Can you work these out from the model? Positions are in its coordinate system, mm. A direction names the side the tool comes from. Give positions to 0.01 mm unless a question says otherwise; leave off trailing zeros. Loops run counter-clockwise (first coordinate to the right, second up) from the corner with the lowest first, then second, coordinate; pieces in that order, holes last. Notation, with made-up numbers: (37.25, 47.5) - (67.25, 47.5) arc R10 ccw to (67.25, 55.5) - close; hole circle Ø2 at (78, 75). An arc over 180 degrees is marked (long way). Answer as a JSON object with one key per item and string values. Group by question number.
Item 1: Which directions (+Z, -Z, +X, -X, +Y, -Y) give clear straight access to the entire face, cutting with the end or side of a thin tool? Please do faces 1 (the flat face through (-42, 25, -45)), 2 (the flat face through (-90, 62, -45)), 3 (the flat face through (-88, 90, -45)).
Item 2: Suppose I cut it at C-C on x = -61. Write out the boundary of the cut face in (y, z), and give its area (3 significant figures).
Item 3: Thinking about a two-plate mould opening in Y: for faces 4 (the flat face through (-72.075, 17.43, -45.49)), 5 (the flat face through (-28, 0, -45)), 6 (the cylindrical face through (-71.014, 84.297, -44.51)), 7 (the flat face through (-66, 34, -80)), which applies, pulls with the +Y half, pulls with the -Y half, needs draft (parallel to the pull), parting line crosses it, or undercut?
Item 4: Will these pins go through, and if not, where does the flat tip stop? pin 1 (6 mm diameter, centred on y = 27.5, z = -28.5, fed in from -X); pin 2 (22.5 mm diameter, centred on y = 45, z = -49, fed in from +X); pin 3 (3 mm diameter, centred on x = -57, z = -50.5, fed in from -Y).
Item 5: Suppose I cut it at B-B on y = 53.5. Write out the boundary of the cut face in (x, z).
Item 6: Suppose I cut it at A-A on z = -45. Write out the boundary of the cut face in (x, y).
Item 7: Suppose I cut it at D-D on y = 10.5. Count the separate pieces of the cut face and the enclosed holes in it, and give its area (3 significant figures).
Item 8: Please list where these lines run through material, in increasing order: L1, parallel to X at y = 66.5, z = -18; L2, parallel to Z at x = -74.5, y = 10.5; L3, parallel to Y at x = -43, z = -56.5.
from build123d import *

# Parameters (mm, degrees)
SKETCH1_W           = 90
SKETCH1_H           = 80
BOSS_EXTRUDE1_DEPTH = 90
SKETCH2_W           = 65
SKETCH2_H           = 65
CUT_EXTRUDE1_DEPTH  = 100
FILLET1_R           = 20
CUT_EXTRUDE2_DEPTH  = 100
SKETCH4_R           = 7.5
BOSS_EXTRUDE2_DEPTH = 150
SKETCH6_W           = 10
SKETCH6_H           = 127.279220614
CUT_EXTRUDE4_DEPTH  = 212.224744882


with BuildPart() as part:
    # Sketch1 → Boss-Extrude1 (new body)
    with BuildSketch(Plane(origin=(0, 0, 0), x_dir=(1, 0, 0), z_dir=(0, 1, 0))):
        with Locations((-45, 40)):
            Rectangle(SKETCH1_W, SKETCH1_H)
    extrude(amount=BOSS_EXTRUDE1_DEPTH)

    # Sketch2 → Cut-Extrude1 (cut)
    with BuildSketch(Plane(origin=(0, 0, -80), x_dir=(-1, 0, 0), z_dir=(0, 0, -1))):
        with Locations((32.5, 57.5)):
            Rectangle(SKETCH2_W, SKETCH2_H)
    extrude(amount=-CUT_EXTRUDE1_DEPTH, mode=Mode.SUBTRACT)

    # Fillet1
    fillet1_edges = [part.edges().sort_by_distance(p)[0] for p in [
        (-65, 90, -40),
        (0, 25, -40),
    ]]
    fillet(fillet1_edges, radius=FILLET1_R)

    # Sketch3 → Cut-Extrude2 (cut)
    with BuildSketch(Plane(origin=(0, 0, -80), x_dir=(-1, 0, 0), z_dir=(0, 0, -1))):
        Polygon((54.644660941, 0), (90, 35.355339059), (90, 0), align=None)
    extrude(amount=-CUT_EXTRUDE2_DEPTH, mode=Mode.SUBTRACT)

    # Sketch4 → Boss-Extrude2 (add)
    with BuildSketch(Plane(origin=(-27.32233047, -27.32233047, 0), x_dir=(0, 0, 1), z_dir=(-0.7071067811865477, -0.7071067811865475, 0))):
        with Locations(Location((-60, 63.639610307, 0), (0, 0, 90))):
            Circle(SKETCH4_R)
        with Locations(Location((-20, 63.639610307, 0), (0, 0, 90))):
            Circle(SKETCH4_R)
    extrude(amount=BOSS_EXTRUDE2_DEPTH)

    # Sketch6 → Cut-Extrude4 (cut, through all)
    with BuildSketch(Plane(origin=(-27.32233047, -27.32233047, 0), x_dir=(0, 0, 1), z_dir=(-0.7071067811865477, -0.7071067811865475, 0))):
        with Locations((-5, 63.639610307)):
            Rectangle(SKETCH6_W, SKETCH6_H)
    extrude(amount=-CUT_EXTRUDE4_DEPTH, mode=Mode.SUBTRACT)


solid = part.part
Worked out:
{
 "1": {"face 1": "+Z, -Z, +X, +Y", "face 2": "+Z, -Z, -X, +Y", "face 3": "+Z, -Z, +X, -X, +Y"},
 "2": {"outline": "(6.36, -80) - (25, -80) - (25, -10) - (6.36, -10) - close", "area": "1,310 mm2"},
 "3": {"face 4": "undercut", "face 5": "pulls with the -Y half", "face 6": "pulls with the +Y half", "face 7": "needs draft"},
 "4": {"pin 1": "stops at x = -85.14", "pin 2": "stops at x = -65", "pin 3": "stops at y = 0.86"},
 "5": {"outline": "(-90, -80) - (-65, -80) - (-65, -10) - (-90, -10) - close"},
 "6": {"outline": "(-90, 35.36) - (-54.64, 0) - (0, 0) - (0, 5) arc R20 ccw to (-20, 25) - (-65, 25) - (-65, 70) arc R20 ccw to (-85, 90) - (-90, 90) - close"},
 "7": {"separate pieces": "3", "enclosed holes": "0", "area": "5,010 mm2"},
 "8": {"L1": "x = -90 to -65", "L2": "z = -66.61 to -53.39, -26.61 to -13.39", "L3": "y = 0 to 25"}
}
